from build123d import *

# Parameters (mm, degrees)
F0_W     = 762
F0_H     = 381
F1_DEPTH = 25.4
F2_R     = 165.1
F3_DEPTH = 12.7
F4_R     = 152.4
F5_DEPTH = 25.4
F7_DEPTH = 762


with BuildPart() as f1:
    # F0 (on Front) → F1 (new body)
    with BuildSketch(Plane.XZ):
        Rectangle(F0_W, F0_H)
    extrude(amount=-F1_DEPTH)

    # F2 (on face) → F3 (cut)
    with BuildSketch(Plane.XZ):
        with Locations((-190.5, 0)):
            Circle(F2_R)
        with Locations((190.5, 0)):
            Circle(F2_R)
    extrude(amount=-F3_DEPTH, mode=Mode.SUBTRACT)

    # F4 (on face) → F5 (cut)
    with BuildSketch(Plane.XZ.offset(-12.7)):
        with Locations((-190.5, 0)):
            Circle(F4_R)
        with Locations((190.5, 0)):
            Circle(F4_R)
    extrude(amount=-F5_DEPTH, mode=Mode.SUBTRACT)

    # F6 (on face) → F7 (cut)
    with BuildSketch(Plane.YZ.offset(381)):
        Polygon((0, -190.5), (25.4, -190.5), (25.4, -152.4), align=None)
        Polygon((25.4, 190.5), (0, 190.5), (25.4, 152.4), align=None)
    extrude(amount=-F7_DEPTH, mode=Mode.SUBTRACT)


solid = f1.part
Model file for the job. Use its own axes, mm. A direction names the side the tool comes from. Give positions to 0.01 mm unless a question says otherwise; leave off trailing zeros. Loops run counter-clockwise (first coordinate to the right, second up) from the corner with the lowest first, then second, coordinate; pieces in that order, holes last.
1) Saw through at C-C (x = 270). Write the cut outline in (y, z), plus the area to 3 significant figures.
2) Saw through at B-B (z = 0). Write the cut outline in (x, y), plus the area to 3 significant figures.
3) Saw through at D-D (z = 54.5). Write the cut outline in (x, y), plus the area to 3 significant figures.
4) Flat gauge pins, fed straight in: pin 1 Ø12 at (x, y) = (189.5, 21) entering from +Z; pin 2 Ø10 at (x, y) = (-269.5, 22) entering from -Z; pin 3 Ø12 at (x, y) = (-294, 6.5) entering from +Z. Where does each tip first touch, or does it go through?
5) Wall check: line 1 (X direction, y = 17.5, z = 0); line 2 (Z direction, x = 190.5, y = 17); line 3 (X direction, y = 23.75, z = 115.5). Give the ranges that are in metal, low to high.
6) Pull direction Z, two halves, no side cores. Call faces 3 (the flat face through (5, 13, -171)), 4 (the cylindrical face through (-226.29, 6.261, -161.174)), 5 (the flat face through (-5, 0, 3)): +Z half, -Z half, draft (parallel to the pull), parting line (faces both ways), or undercut.
7) Saw through at A-A (y = 8.5). Write the cut outline in (x, z), plus the area to 3 significant figures.
8) Tool access for faces 1 (the flat face through (239, 12.7, -146)), 2 (the cylindrical face through (331.28, 18.96, -58.37)): list every direction of +Z, -Z, +X, -X, +Y, -Y with a clear straight run to the whole face (end or side of a thin tool).
Answer block:
1. outline: (0, -190.5) - (25.4, -152.4) - (25.4, -130.02) - (12.7, -130.02) - (12.7, -144.7) - (0, -144.7) - close; (0, 144.7) - (12.7, 144.7) - (12.7, 130.02) - (25.4, 130.02) - (25.4, 152.4) - (0, 190.5) - close
1. area: 1,730 mm2
2. outline: (-381, 0) - (-355.6, 0) - (-355.6, 12.7) - (-342.9, 12.7) - (-342.9, 25.4) - (-381, 25.4) - close; (-38.1, 12.7) - (-25.4, 12.7) - (-25.4, 0) - (25.4, 0) - (25.4, 12.7) - (38.1, 12.7) - (38.1, 25.4) - (-38.1, 25.4) - close; (342.9, 12.7) - (355.6, 12.7) - (355.6, 0) - (381, 0) - (381, 25.4) - (342.9, 25.4) - close
2. area: 3,230 mm2
3. outline: (-381, 0) - (-346.35, 0) - (-346.35, 12.7) - (-332.82, 12.7) - (-332.82, 25.4) - (-381, 25.4) - close; (-48.18, 12.7) - (-34.65, 12.7) - (-34.65, 0) - (34.65, 0) - (34.65, 12.7) - (48.18, 12.7) - (48.18, 25.4) - (-48.18, 25.4) - close; (332.82, 12.7) - (346.35, 12.7) - (346.35, 0) - (381, 0) - (381, 25.4) - (332.82, 25.4) - close
3. area: 4,210 mm2
4. pin 1: stops at z = 168
4. pin 2: stops at z = -165
4. pin 3: stops at z = 189.75
5. line 1: x = -381 to -342.9, -38.1 to 38.1, 342.9 to 381
5. line 2: z = -165 to -152.4, 152.4 to 165
5. line 3: x = -381 to -289.93, -91.07 to 91.07, 289.93 to 381
6. face 3: -Z half
6. face 4: undercut
6. face 5: draft
7. outline: (-381, -177.75) - (381, -177.75) - (381, 177.75) - (-381, 177.75) - close; hole circle Ø330.2 at (-190.5, 0); hole circle Ø330.2 at (190.5, 0)
7. area: 99,600 mm2
8. face 1: -Y
8. face 2: +Y, -Y
